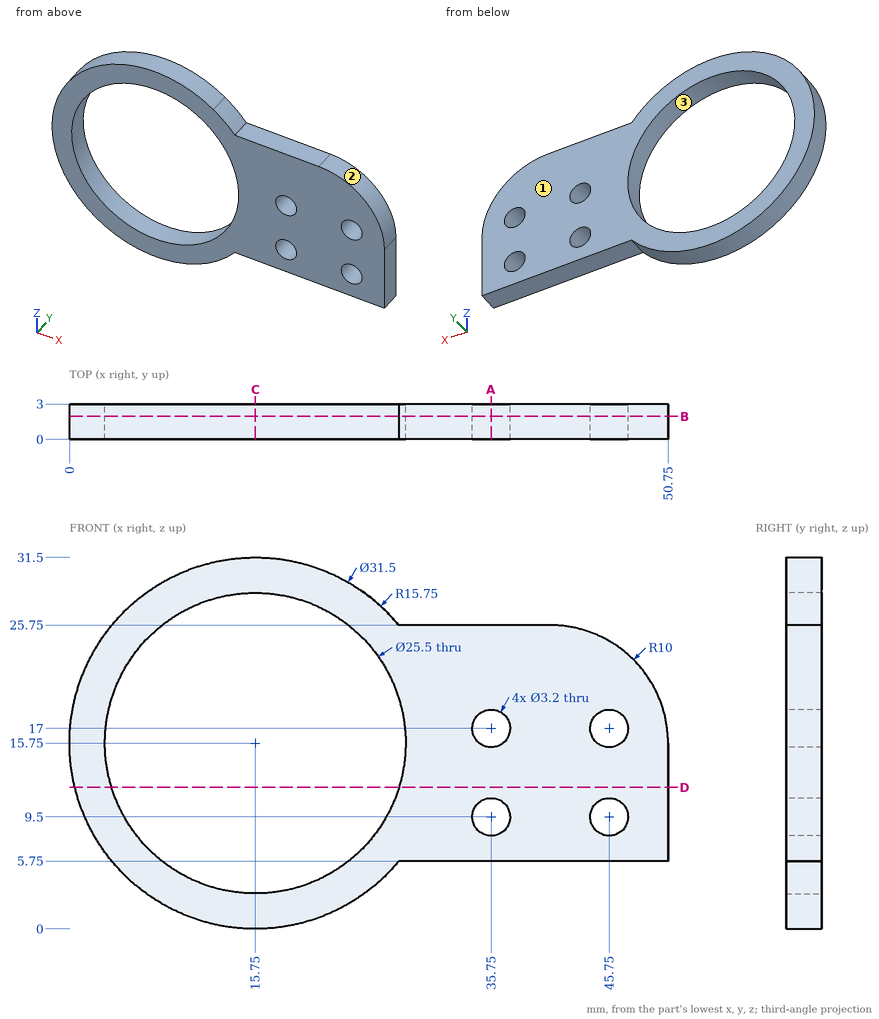
Answer from the drawing. Dimensions are ordinates in mm from the lowest x, y and z of the part. Coordinates: 2 decimals unless noted, no trailing zeros. Loops run counter-clockwise (first coordinate to the right, second up) from the corner with the lowest first, then second, coordinate; pieces in that order, holes last. Notation, with made-up numbers: (2, 87.25) -> (39, 87.25) arc R12 ccw to (39, 106.25) -> close; hole circle Ø7 at (-38, -32). An arc over 180 degrees is marked (long way). Answer in a Markdown table with one row per item.
Item 1: A cutting plane is placed at B-B on y = 1.95. Determine the outline of the cut face in (x, z), plus the area to 3 significant figures.
Returned:
| item | result |
|---|---|
| outline | (27.92, 5.75) -> (50.75, 5.75) -> (50.75, 15.75) arc R10 ccw to (40.75, 25.75) -> (27.92, 25.75) arc R15.75 ccw (long way) to start; hole circle Ø25.5 at (15.75, 15.75); hole circle Ø3.2 at (35.75, 9.5); hole circle Ø3.2 at (35.75, 17); hole circle Ø3.2 at (45.75, 9.5); hole circle Ø3.2 at (45.75, 17) |
| area | 623 mm^2 |
Item 2: Each of these flat-tipped pins is pushed along its axis until it touches: P1, Ø3.5, axis at x = 35.75, z = 17, coming from the -Y side; P2, Ø1.5, axis at y = 0.5, z = 22.5, coming from the -X side. Where does it stop, or does it pass through?
Returned:
| item | result |
|---|---|
| P1 | stops at y = 0 |
| P2 | stops at x = 1.19 |
Item 3: A cutting plane is placed at D-D on z = 12. Determine the outline of the cut face in (x, y).
Returned:
| item | result |
|---|---|
| outline | (0.45, 0) -> (3.56, 0) -> (3.56, 3) -> (0.45, 3) -> close; (27.94, 0) -> (50.75, 0) -> (50.75, 3) -> (27.94, 3) -> close |
Item 4: Straight lines are drawn through the part: line 1 along X through (y, z) = (1.25, 17); line 2 along X through (y, z) = (1.2, 16.5); line 3 along X through (y, z) = (0.85, 4.5). For each, find the intervals that lie inside material, in ascending order. Write a range as [from, to].
Returned:
| item | result |
|---|---|
| line 1 | x = [0.05, 3.06], [28.44, 34.15], [37.35, 44.15], [47.35, 50.67] |
| line 2 | x = [0.02, 3.02], [28.48, 34.23], [37.27, 44.23], [47.27, 50.72] |
| line 3 | x = [4.73, 9.75], [21.75, 26.77] |
Item 5: For a pull along Z with two mould halves and no side action, classify the marked faces 1, 2 and 3 as released by +Z, released by -Z, zero draft, split by the parting line, or undercut.
Returned:
| item | result |
|---|---|
| face 1 | zero draft |
| face 2 | released by +Z |
| face 3 | undercut |
Item 6: A cutting plane is placed at C-C on x = 15.75. Determine the outline of the cut face in (y, z).
Returned:
| item | result |
|---|---|
| outline | (0, 0) -> (3, 0) -> (3, 3) -> (0, 3) -> close; (0, 28.5) -> (3, 28.5) -> (3, 31.5) -> (0, 31.5) -> close |
Item 7: A cutting plane is placed at A-A on x = 35.75. Determine the outline of the cut face in (y, z), plus the area to 3 significant figures.
Returned:
| item | result |
|---|---|
| outline | (0, 5.75) -> (3, 5.75) -> (3, 7.9) -> (0, 7.9) -> close; (0, 11.1) -> (3, 11.1) -> (3, 15.4) -> (0, 15.4) -> close; (0, 18.6) -> (3, 18.6) -> (3, 25.75) -> (0, 25.75) -> close |
| area | 40.8 mm^2 |
